Source: CAD feature listing. Evaluate the final solid. Frame: model axes, mm. A direction names the side the tool comes from. Round coordinates to 2 decimals unless told otherwise and drop trailing zeros. Order: outer loops, then holes, each group sorted by start corner. A loop starts at its lowest first (then second) coordinate and runs counter-clockwise, first axis right, second up. Notation, with made-up numbers: M 53.5,23 L 102.5,23 A32 ccw 102.5,59 Z; hole C 25.25,-8.75 d1. An arc over 180 degrees is marked long. Use one line per item in the form item = value. Start each with the question number.
Q1. Reachability of faces 4 (the flat face through (33, 52, 28)), 5 (the flat face through (-26, 7, 10)), 6 (the cylindrical face through (-12.702, -9.7, -0.675)), 7 (the flat face through (30.833, 52, 11)), 8 (the flat face through (33, 47.258, 24)) from +Z, -Z, +X, -X, +Y, -Y: full face, straight path, thin tool, end or side. Return the list, or none.
Q2. Section C-C (y = 32.5). Return the cut outline in (x, z), plus the area to 3 significant figures.
Q3. Section A-A (z = 23). Return the cut outline in (x, y).
Q4. Material intervals for probe 1 along X at (y, z) = (-9.85, -1); probe 2 along Y at (x, z) = (32.15, -1); probe 3 along Y at (x, z) = (-26, 5), sorted ascending.
Q5. Pull-direction query (Z, two-part tool) for faces 1 (the cylindrical face through (-5.654, -9.7, -0.805)), 2 (the flat face through (-22.167, 10, 2)), 3 (the flat face through (-25.62, 24.79, 7.47)); classes: pulls with the +Z half, pulls with the -Z half, needs draft (parallel to the pull), parting line crosses it, or undercut.
Q6. Contact query for flat-ended pins moving along their axis: pin 1 (1.8 mm diameter, centred on y = 52.26, z = -1, fed in from -X); pin 2 (8 mm diameter, centred on x = 21.5, z = 5.5, fed in from -Y); pin 3 (5.5 mm diameter, centred on x = -27, y = 5.5, fed in from +Z); pin 4 (4 mm diameter, centred on y = 52.26, z = 23, fed in from +X). Output: stop coordinate, or through.
Q7. Section D-D (x = 4.5). Return the cut outline in (y, z), plus the area to 3 significant figures.
Q8. Section B-B (y = 16). Return the cut outline in (x, z), plus the area to 3 significant figures.
Autodesk Inventor part; units mm, degrees
ref_plane "YZ Plane" through (0, 0, 0) normal (1, 0, 0) x (0, 1, 0)
ref_plane "XZ Plane" through (0, 0, 0) normal (0, 1, 0) x (-1, 0, 0)
ref_plane "XY Plane" through (0, 0, 0) normal (0, 0, 1) x (1, 0, 0)
sketch "Sketch1" plane through (0, 0, 0) normal (0, 0, 1) x (1, 0, 0)
  line L0 (-29.1667, 27.2576) -> (-22.1667, 27.2576)
  line L1 (-22.1667, 27.2576) -> (-22.1667, -12.7424)
  line L2 (-22.1667, -12.7424) -> (-29.1667, -12.7424)
  line L3 (-29.1667, -12.7424) -> (-29.1667, 27.2576)
  point P0 (0, 0)
  dimension "d0" = 7
  dimension "d1" = 40
extrude "Extrusion1" add sketch "Sketch1" along normal blind 10
sketch "Sketch2" plane through (-22.1667, -12.7424, 0) normal (1, 0, 0) x (0, 0, -1)
  line L0 (-10, 0) -> (-10, 40)
  line L1 (0, 40) -> (-10, 40)
  point P0 (0, 12.7424)
  point P1 (-5, 35)
  dimension "d4" = 5
  dimension "d5" = 5
hole "Hole1" at (-22.1667, 22.2576, 5) direction (-1, 0, 0) diameter 3 depth 8 tip angle 118 countersink diameter 6 countersink angle 90
sketch "Sketch3" plane through (0, 0, 10) normal (0, 0, 1) x (1, 0, 0)
  line L0 (-29.1667, -12.7424) -> (30.8333, -12.7424)
  line L1 (30.8333, -12.7424) -> (30.8333, -8.7424)
  line L2 (30.8333, -8.7424) -> (-29.1667, -8.7424)
  line L3 (-29.1667, -8.7424) -> (-29.1667, -12.7424)
  line L4 (30.8333, -12.7424) -> (26.8333, -12.7424)
  line L5 (26.8333, -12.7424) -> (26.8333, 52.2576)
  line L6 (26.8333, 52.2576) -> (30.8333, 52.2576)
  line L7 (30.8333, 52.2576) -> (30.8333, -12.7424)
  point P0 (0, 0)
  dimension "d13" = 60
  dimension "d14" = 4
  dimension "d15" = 4
  dimension "d16" = 65
extrude "Extrusion2" add sketch "Sketch3" against normal blind 10
sketch "Sketch4" plane through (30.8333, 52.2576, 10) normal (1, 0, 0) x (0, 0, -1)
  line L0 (16, -5) -> (-18, -5)
  line L1 (-18, -5) -> (-18, 5)
  line L2 (-18, 5) -> (16, 5)
  line L3 (16, 5) -> (16, -5)
  line L4 (0, 0) -> (10, 0)
  circle A0 centre (5, -30) radius 1.5
  point P0 (10, -52.2576)
  dimension "d21" = 5
  dimension "d22" = 23
  dimension "d23" = 11
  dimension "d24" = 5
extrude "Extrusion3" add sketch "Sketch4" against normal blind 4 contours L0 L1 L2 L3
sketch "Sketch9" plane through (0, 0, 10) normal (0, 0, 1) x (1, 0, 0)
  line L0 (26.7106, 42.2576) -> (30.8333, 47.2576)
  line L1 (30.8333, 47.2576) -> (34.8333, 47.2576)
  line L2 (34.8333, 47.2576) -> (30.8333, 47.2576)
  line L3 (34.8333, 47.2576) -> (30.7106, 42.2576)
  line L4 (30.7106, 42.2576) -> (26.7106, 42.2576)
  point P0 (0, 0)
extrude "Extrusion8" add sketch "Sketch9" against normal blind 10
sketch "Sketch10" plane through (0, 0, 10) normal (0, 0, 1) x (1, 0, 0)
  line L0 (30.8333, 42.2576) -> (34.8333, 47.2576)
  line L1 (34.8333, 47.2576) -> (34.8333, 42.2576)
  line L2 (30.8333, 47.2576) -> (34.8333, 47.2576)
  line L3 (34.8333, 42.2576) -> (30.8333, 42.2576)
  point P0 (0, 0)
extrude "Extrusion9" cut sketch "Sketch10" against normal blind 10
sketch "Sketch12" plane through (0, 0, 0) normal (0, 0, -1) x (-1, 0, 0)
  point P0 (0, 0)
sketch "Sketch13" plane through (0, 0, 0) normal (0, 0, -1) x (-1, 0, 0)
  line L0 (29.1667, -12.7424) -> (-30.8333, -12.7424)
  line L1 (-30.8333, -12.7424) -> (-30.8333, -8.7424)
  line L2 (-30.8333, -8.7424) -> (29.1667, -8.7424)
  line L3 (29.1667, -8.7424) -> (29.1667, -12.7424)
  line L4 (-30.8333, 42.2576) -> (-26.8333, 42.2576)
  line L5 (-26.8333, 42.2576) -> (-26.8333, -12.7424)
  line L6 (-26.8333, -12.7424) -> (-30.8333, -12.7424)
  line L7 (-30.8333, -12.7424) -> (-30.8333, 42.2576)
  line L8 (-30.8333, 42.2576) -> (-34.8333, 47.2576)
  line L9 (-34.8333, 47.2576) -> (-30.8333, 42.2576)
  line L10 (-34.8333, 47.2576) -> (-30.8333, 47.2576)
  line L11 (-30.8333, 47.2576) -> (-26.8333, 42.2576)
  point P0 (0, 0)
  dimension "d53" = 60
  dimension "d54" = 4
  dimension "d55" = 4
extrude "Extrusion10" add sketch "Sketch13" along normal blind 6
sketch "Sketch14" plane through (0, 0, 10) normal (0, 0, 1) x (1, 0, 0)
  point P0 (0, 0)
sketch "Sketch15" plane through (0, 0, 10) normal (0, 0, 1) x (1, 0, 0)
  line L0 (-29.1667, -12.7424) -> (30.8333, -12.7424)
  line L1 (34.8333, 47.2576) -> (-22.1667, 47.2576)
  line L2 (-22.1667, 47.2576) -> (-22.1667, -12.7424)
  line L3 (-22.1667, -12.7424) -> (34.8333, -12.7424)
  line L4 (34.8333, -12.7424) -> (34.8333, 47.2576)
  line L5 (-22.1667, -8.7424) -> (-22.1667, 27.2576)
  point P0 (0, 0)
extrude "Extrusion11" cut sketch "Sketch15" against normal blind 20
sketch "Sketch16" plane through (0, 0, -6) normal (0, 0, -1) x (-1, 0, 0)
  line L0 (29.1667, -12.7424) -> (-30.8333, -12.7424)
  line L1 (-30.8333, -12.7424) -> (-30.8333, -8.7424)
  line L2 (-30.8333, -8.7424) -> (29.1667, -8.7424)
  line L3 (29.1667, -8.7424) -> (29.1667, -12.7424)
  line L4 (-30.8333, 47.2576) -> (-26.8333, 47.2576)
  line L5 (-26.8333, 47.2576) -> (-26.8333, -12.7424)
  line L6 (-26.8333, -12.7424) -> (-30.8333, -12.7424)
  line L7 (-30.8333, -12.7424) -> (-30.8333, 47.2576)
  line L8 (-30.8333, 57.2576) -> (-30.8333, 47.2576)
  point P0 (0, 0)
  dimension "d60" = 4
  dimension "d61" = 4
extrude "Extrusion12" add sketch "Sketch16" against normal blind 20
sketch "Sketch17" plane through (0, 0, 0) normal (0, 0, -1) x (-1, 0, 0)
  line L0 (29.1667, 27.2576) -> (22.1667, 27.2576)
  line L1 (22.1667, 27.2576) -> (22.1667, -8.7424)
  line L2 (22.1667, -8.7424) -> (29.1667, -8.7424)
  line L3 (29.1667, -8.7424) -> (29.1667, 27.2576)
  point P0 (0, 0)
extrude "Extrusion13" add sketch "Sketch17" along normal blind 6
sketch "Sketch18" plane through (30.8333, 47.2576, 28) normal (1, 0, 0) x (0, 0, -1)
  line L0 (0, 0) -> (0, 10)
  line L1 (34, 10) -> (34, -60)
  point P0 (28, -47.2576)
  point P1 (5, 5)
  point P2 (29, 5)
  dimension "d66" = 5
  dimension "d67" = 5
hole "Hole3" at (30.8333, 52.2576, 23) at (30.8333, 52.2576, -1) direction (-1, 0, 0) diameter 3 depth 8 tip angle 118 countersink diameter 6 countersink angle 90
fillet "Fillet4" radius 55 2 edges at (26.8333, -8.7424, 4) (30.8333, -12.7424, 4)
chamfer "Chamfer2" distance 4 angle 45 1 edges at (-29.1667, -10.7424, 14)
chamfer "Chamfer3" distance 5 angle 45 2 edges at (28.8333, 47.2576, 14) (-25.6667, 27.2576, 10)
sketch "Sketch19" plane through (30.8333, 47.2576, 28) normal (1, 0, 0) x (0, 0, -1)
  line L0 (0, 0) -> (34, 0)
  line L1 (34, 0) -> (34, 10)
  line L2 (34, 10) -> (0, 10)
  line L3 (0, 10) -> (0, 0)
  point P0 (28, -47.2576)
extrude "Extrusion14" add sketch "Sketch19" along normal blind 4
sketch "Sketch20" plane through (30.8333, 42.2576, -6) normal (1, 0, 0) x (0, 0, -1)
  line L0 (-20, 0) -> (0, 0)
  line L1 (0, 0) -> (0, 5)
  line L2 (0, 5) -> (-20, 5)
  line L3 (-20, 5) -> (-20, 0)
  point P0 (-6, -42.2576)
extrude "Extrusion15" add sketch "Sketch20" along normal blind 4
chamfer "Chamfer4" distance 5 angle 45 1 edges at (32.8333, 47.2576, 14)
sketch "Sketch21" plane through (26.8333, 47.2576, 28) normal (-1, 0, 0) x (0, 0, 1)
  line L0 (-34, -5) -> (-34, 10)
  line L1 (0, 10) -> (-34, 10)
  line L2 (-34, 10) -> (-34, 0)
  line L3 (-34, 0) -> (0, 0)
  line L4 (0, 0) -> (0, 10)
  line L5 (-9, 0) -> (0, 0)
  point P0 (-28, -47.2576)
extrude "Extrusion16" cut sketch "Sketch21" against normal blind 4
chamfer "Chamfer5" distance 1 angle 45 1 edges at (26.8333, 47.2576, 6.5)
sketch "Sketch22" plane through (34.8333, 47.2576, 28) normal (1, 0, 0) x (0, 0, -1)
  line L0 (0, 10) -> (0, 0)
  line L1 (34, 10) -> (0, 10)
  line L2 (34, -5) -> (34, 10)
  point P0 (28, -47.2576)
  point P1 (5, 5)
  point P2 (29, 5)
  dimension "d94" = 5
  dimension "d95" = 5
  dimension "d96" = 5
  dimension "d97" = 5
hole "Hole4" at (34.8333, 52.2576, 23) at (34.8333, 52.2576, -1) direction (-1, 0, 0) diameter 3 depth 8 tip angle 118 countersink diameter 6 countersink angle 90
sketch "Sketch23" plane through (30.8333, 47.2576, 19) normal (0, 1, 0) x (1, 0, 0)
  line L0 (0, 0) -> (-4, 0)
  line L1 (-4, 0) -> (-4, 25)
  line L2 (-4, 25) -> (0, 25)
  line L3 (0, 25) -> (0, 0)
  point P0 (-30.8333, 19)
extrude "Extrusion17" cut sketch "Sketch23" against normal blind 1
sketch "Sketch24" plane through (0, 0, 10) normal (0, 0, 1) x (1, 0, 0)
  point P0 (0, 0)
ref_plane "Work Plane1" through (15.8333, -12.7424, -6) normal (-1, 0, 0) x (0, 0, 1)
sketch "Sketch25" plane through (15.8333, -12.7424, -6) normal (-1, 0, 0) x (0, 0, 1)
  circle A0 centre (11, 35) radius 1.5
  circle A1 centre (11, 35) radius 5
  point P0 (6, 12.7424)
  dimension "d108" = 10
extrude "Extrusion18" cut sketch "Sketch25" against normal blind 50 contours A0 | A1
sketch "Sketch26" plane through (0, 0, 14) normal (0, 0, 1) x (1, 0, 0)
  line L0 (-24.1667, -12.7424) -> (0.8333, -12.7424)
  line L1 (0.8333, -12.7424) -> (0.8333, -8.7424)
  line L2 (0.8333, -8.7424) -> (-24.1667, -8.7424)
  line L3 (-24.1667, -8.7424) -> (-24.1667, -12.7424)
  line L4 (0.8333, -8.7424) -> (-4.1667, -8.7424)
  line L5 (-4.1667, -8.7424) -> (-4.1667, -5.7424)
  line L6 (-4.1667, -5.7424) -> (0.8333, -5.7424)
  line L7 (0.8333, -5.7424) -> (0.8333, -8.7424)
  point P0 (0, 0)
  dimension "d111" = 25
  dimension "d112" = 4
  dimension "d113" = 5
  dimension "d114" = 3
extrude "Extrusion19" add sketch "Sketch26" against normal blind 20
sketch "Sketch27" plane through (-29.1667, -12.7424, -6) normal (0, -1, 0) x (1, 0, 0)
  line L0 (55.8544, 20) -> (4, 20)
  line L1 (30, 20) -> (30, 0)
  line L2 (30, 0) -> (0, 0)
  point P0 (29.1667, 6)
  point P1 (25, 15)
  point P2 (25, 5)
  point P3 (15, 5)
  dimension "d117" = 5
  dimension "d118" = 5
  dimension "d119" = 5
  dimension "d120" = 5
  dimension "d121" = 10
hole "Hole5" at (-4.1667, -12.7424, 9) at (-4.1667, -12.7424, -1) at (-14.1667, -12.7424, -1) direction (0, 1, 0) diameter 3 depth 6 tip angle 118
sketch "Sketch28" plane through (-29.1667, -12.7424, -6) normal (0, -1, 0) x (1, 0, 0)
  line L0 (8.7267, 12.1008) -> (6.2978, 10.7688)
  line L1 (6.2978, 10.7688) -> (8.7267, 9.2201)
  line L2 (8.7267, 9.2201) -> (8.7267, 12.1008)
  point P0 (29.1667, 6)
extrude "Extrusion20" cut sketch "Sketch28" against normal blind 1
properties part number "z-stepper support arm"
Results list:
q1.face_4 = +Z, +X, -X, +Y, -Y
q1.face_5 = +Z, -X, +Y
q1.face_6 = -Y
q1.face_7 = +Z, -Z, -X, +Y
q1.face_8 = +Z, +X, -X, -Y
q2.outline = M 25.08,-6 L 29.96,-6 L 29.96,14 L 25.08,14 Z
q2.area = 97.5 mm2
q3.outline = M 30.83,47.26 L 34.83,47.26 L 34.83,49.26 L 33.33,50.76 L 30.83,50.76 Z; M 30.83,53.76 L 33.33,53.76 L 34.83,55.26 L 34.83,57.26 L 30.83,57.26 Z
q4.probe_1 = -29.17 to -15.67, -12.67 to -5.67, -2.67 to 0.83
q4.probe_2 = 42.26 to 50.76, 53.76 to 57.26
q4.probe_3 = -12.74 to 20.76, 23.76 to 27.26
q5.face_1 = undercut
q5.face_2 = needs draft
q5.face_3 = pulls with the +Z half
q6.pin_1 = through
q6.pin_2 = 6.36
q6.pin_3 = 10
q6.pin_4 = 33.84
q7.outline = M -4.68,-6 L 2.01,-6 L 2.01,14 L -4.68,14 Z
q7.area = 134 mm2
q8.outline = M -29.17,-6 L -22.17,-6 L -22.17,10 L -29.17,10 Z; M 17.76,-6 L 24.16,-6 L 24.16,14 L 17.76,14 Z
q8.area = 240 mm2
